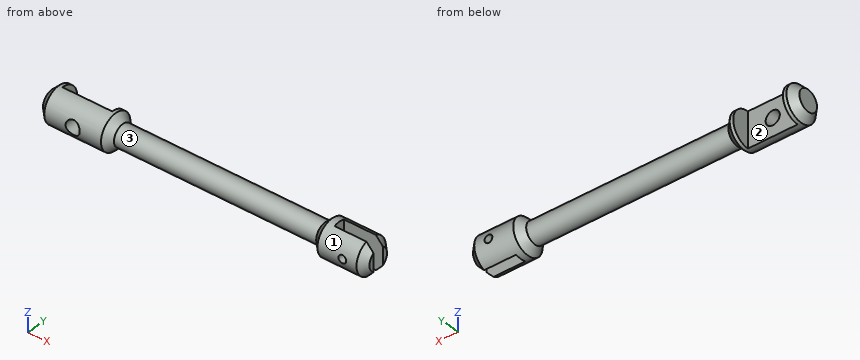
```python
from build123d import *

# Parameters (mm, degrees)
F2_DEPTH = 12.7
F3_W     = 7
F3_H     = 4.492721
F3_W_2   = 5.5
F3_H_2   = 1.6
F4_DEPTH = 12.7


with BuildPart() as f1:
    # F0 (on Front) → F1 (revolve)
    with BuildSketch(Plane.XZ):
        with BuildLine():
            ThreePointArc((-1, 0), (0, 1), (1, 0))
            Line((1, 0), (37.45, 0))
            ThreePointArc((37.45, 0), (38, 0.55), (38.55, 0))
            Line((38.55, 0), (41, 0))
            Line((41, 0), (41, 1.5))
            Line((41, 1.5), (40, 2.5))
            Line((40, 2.5), (34.5, 2.5))
            Line((34.5, 2.5), (33.5, 1.5))
            Line((33.5, 1.5), (5, 1.5))
            Line((5, 1.5), (4, 2.5))
            Line((4, 2.5), (-4, 2.5))
            Line((-4, 2.5), (-5, 1.5))
            Line((-5, 1.5), (-5, 0))
            Line((-5, 0), (-1, 0))
        make_face()
        with BuildLine():
            ThreePointArc((-1, 0), (0, -1), (1, 0))
            Line((1, 0), (-1, 0))
        make_face()
        with BuildLine():
            Line((38.55, 0), (37.45, 0))
            ThreePointArc((37.45, 0), (38, -0.55), (38.55, 0))
        make_face()
    revolve(axis=Axis((18, 0, 0), (1, 0, 0)))

    # F0 (on Front) → F2 (cut, symmetric)
    with BuildSketch(Plane.XZ):
        with BuildLine():
            Line((-1, 0), (1, 0))
            ThreePointArc((1, 0), (0, 1), (-1, 0))
        make_face()
        with BuildLine():
            ThreePointArc((-1, 0), (0, -1), (1, 0))
            Line((1, 0), (-1, 0))
        make_face()
        with BuildLine():
            ThreePointArc((38.55, 0), (38, 0.55), (37.45, 0))
            Line((37.45, 0), (38.55, 0))
        make_face()
        with BuildLine():
            Line((38.55, 0), (37.45, 0))
            ThreePointArc((37.45, 0), (38, -0.55), (38.55, 0))
        make_face()
    extrude(amount=F2_DEPTH, both=True, mode=Mode.SUBTRACT)

    # F3 (on Top) → F4 (cut, symmetric)
    with BuildSketch(Plane.XY):
        with Locations((0, 2.24636)):
            Rectangle(F3_W, F3_H)
        with Locations((38.25, 0)):
            Rectangle(F3_W_2, F3_H_2)
    extrude(amount=F4_DEPTH, both=True, mode=Mode.SUBTRACT)


solid = f1.part
```
Check sheet for the modelled part. Datum: model origin and axes. Units: mm. Face numbers are marked on the shaded views. A direction names the side the tool comes from. Round coordinates to 2 decimals unless told otherwise and drop trailing zeros. Write each loop counter-clockwise with the first axis right and the second up, starting at its lowest first coordinate (ties: lowest second). Pieces come first, ordered by that corner, then holes. Notation, with made-up numbers: M 39.25,29 L 52.25,29 A17 ccw 52.25,61 Z; hole C 20.25,55 d11. An arc over 180 degrees is marked long. Write item = value, one per line. Start each with the question number.
1. Section check B-B, the plane y = 2. State how many separate pieces and enclosed holes the cut face has, then the cut area to 3 significant figures.
2. Tool access check on the marked faces 1, 2 and 3. Record the directions out of +Z, -Z, +X, -X, +Y, -Y that give a thin tool (end or side, any length) a straight path to the whole face; none if there is none.
3. Section check A-A, the plane x = 36.5. Record the cut outline in (y, z).
4. Gauge pin test, flat ends, axial feed: pin 1 (1.4 mm diameter, centred on x = 38.5, z = 1, fed in from -Y); pin 2 (2 mm diameter, centred on x = 20, y = 1, fed in from -Z); pin 3 (2 mm diameter, centred on x = 19.5, z = 1, fed in from -Y). Record the tip position at first contact, or that the pin passes through.
5. Section check D-D, the plane x = 8.5. Record the cut outline in (y, z).
6. Scan lines: line 1 (X direction, y = 0.35, z = -0.9); line 2 (X direction, y = -1.75, z = 0.6); line 3 (X direction, y = -2.15, z = 0.25). Record each from-to range of solid material in increasing order. Write a range as [from, to].
Results found:
q1.separate_pieces = 3
q1.enclosed_holes = 1
q1.area = 22.5 mm^2
q2.face_1 = +X, -X
q2.face_2 = +Z, -Z, +Y
q2.face_3 = none
q3.outline = M -0.8,-2.37 L -0.8,2.37 A2.5 ccw Z; M 0.8,-2.37 A2.5 ccw 0.8,2.37 Z
q4.pin_1 = -2.48
q4.pin_2 = -1.5
q4.pin_3 = -1.5
q5.outline = C 0,0 d3
q6.line_1 = [-5, -3.5], [3.5, 35.5]
q6.line_2 = [-4.65, -0.8], [0.8, 4.65], [33.85, 40.65]
q6.line_3 = [-4.34, -0.97], [0.97, 4.34], [34.16, 37.51], [38.49, 40.34]
